```python
from build123d import *

# Parameters (mm, degrees)
SKETCH1_W               = 123
SKETCH1_H               = 20
SKETCH1_R               = 4.1
SKETCH1_R_2             = 4.5
BOSS_EXTRUDE1_DEPTH     = 8
FILLET1_R               = 5
FILLET2_R               = 5
CUT_EXTRUDE1_REACH      = 126.872
CUT_EXTRUDE1_END_RADIUS = 4.1
SKETCH2_R               = 1.5
CUT_EXTRUDE2_REACH      = 126.872
CUT_EXTRUDE2_END_RADIUS = 4.1
SKETCH3_R               = 1.5


with BuildPart() as part:
    # Sketch1 → Boss-Extrude1 (new body)
    with BuildSketch(Plane.XY):
        with Locations((-61.5, 10)):
            Rectangle(SKETCH1_W, SKETCH1_H)
        with Locations((-113.75, 10)):
            Circle(SKETCH1_R, mode=Mode.SUBTRACT)
        with Locations((-61.5, 10)):
            Circle(SKETCH1_R_2, mode=Mode.SUBTRACT)
        with Locations((-9.25, 10)):
            Circle(SKETCH1_R, mode=Mode.SUBTRACT)
    extrude(amount=BOSS_EXTRUDE1_DEPTH)

    # Fillet1
    fillet1_edges = [part.edges().sort_by_distance(p)[0] for p in [
        (-123, 20, 4),
    ]]
    fillet(fillet1_edges, radius=FILLET1_R)

    # Fillet2
    fillet2_edges = [part.edges().sort_by_distance(p)[0] for p in [
        (0, 0, 4),
        (-123, 0, 4),
        (0, 20, 4),
    ]]
    fillet(fillet2_edges, radius=FILLET2_R)

    # Cut-Extrude1: up to this cylinder (the profile starts outside it)
    cut_extrude1_end = Plane(origin=(-113.75, 10, 4), z_dir=(0, 0, -1)) * Cylinder(CUT_EXTRUDE1_END_RADIUS, 262.944, mode=Mode.PRIVATE)
    # Sketch2 → Cut-Extrude1 (cut, up to the surface)
    with BuildSketch(Plane.ZY.offset(123), mode=Mode.PRIVATE) as cut_extrude1_sk1:
        with Locations((4, 10)):
            Circle(SKETCH2_R)
    cut_extrude1_tool1 = extrude(cut_extrude1_sk1.sketch, amount=-CUT_EXTRUDE1_REACH, mode=Mode.PRIVATE) - cut_extrude1_end
    add(cut_extrude1_tool1.solids().sort_by_distance((-123, 10, 4))[0], mode=Mode.SUBTRACT)

    # Cut-Extrude2: up to this cylinder (the profile starts outside it)
    cut_extrude2_end = Plane(origin=(-9.25, 10, 4), z_dir=(0, 0, -1)) * Cylinder(CUT_EXTRUDE2_END_RADIUS, 262.944, mode=Mode.PRIVATE)
    # Sketch3 → Cut-Extrude2 (cut, up to the surface)
    with BuildSketch(Plane(origin=(0, 0, 0), x_dir=(0, 0, -1), z_dir=(1, 0, 0)), mode=Mode.PRIVATE) as cut_extrude2_sk1:
        with Locations(Location((-4, 10, 0), (0, 0, 180))):
            Circle(SKETCH3_R)
    cut_extrude2_tool1 = extrude(cut_extrude2_sk1.sketch, amount=-CUT_EXTRUDE2_REACH, mode=Mode.PRIVATE) - cut_extrude2_end
    add(cut_extrude2_tool1.solids().sort_by_distance((0, 10, 4))[0], mode=Mode.SUBTRACT)


solid = part.part
```
Geometry check sheet. Reference: the model listing, model coordinates, mm. A direction names the side the tool comes from. Give positions to 0.01 mm unless a question says otherwise; leave off trailing zeros. Order: outer loops, then holes, each group sorted by start corner. A loop starts at its lowest first (then second) coordinate and runs counter-clockwise, first axis right, second up. Notation, with made-up numbers: (-6.5, 57.5) - (21.5, 57.5) arc R11 ccw to (21.5, 71.5) - close; hole circle Ø10 at (-11.75, -8.75). An arc over 180 degrees is marked (long way). Answer in a Markdown table with one row per item. Add a question column.
Q1. Gauge pin test, flat ends, axial feed: pin 1 (2.5 mm diameter, centred on y = 10, z = 4, fed in from +X); pin 2 (4 mm diameter, centred on y = 17.5, z = 4.5, fed in from +X); pin 3 (1.8 mm diameter, centred on y = 10, z = 4, fed in from -X). Record the tip position at first contact, or that the pin passes through.
Q2. Material ranges on probe 1 along Z at (x, y) = (-119.9, 10); probe 2 along X at (y, z) = (8.5, 1); probe 3 along Y at (x, z) = (-113.75, 3.25), recorded low to high. Write a range as from..to.
Q3. Cross-section at D-D, the plane x = -61.5. Enter the section's corners in (y, z), then the cut area to 3 significant figures.
Q4. Mould release check, pull along X, two halves, no side actions. Record for faces 3 (the cylindrical face through (-109.84, 11.23, 3.94)), 4 (the cylindrical face through (-2.679, 10.575, 5.386)), 5 (the cylindrical face through (-2, 1, 4)): pulls with the +X half, pulls with the -X half, needs draft (parallel to the pull), parting line crosses it, or undercut.
Q5. Cross-section at A-A, the plane y = 10. Enter the section's corners in (x, z), then the cut area to 3 significant figures.
Q6. Tool access check on faces 1 (the flat face through (-62, 15, 8)), 2 (the cylindrical face through (-120.321, 9.425, 5.386)). Record the directions out of +Z, -Z, +X, -X, +Y, -Y that give a thin tool (end or side, any length) a straight path to the whole face; none if there is none.
Q7. Cross-section at B-B, the plane z = 1.5. Enter the section's corners in (x, y).
Q8. Cross-section at C-C, the plane x = -113.75. Enter the section's corners in (y, z).
Check values:
| question | item | result |
|---|---|---|
| 1 | pin 1 | stops at x = -13.15 |
| 1 | pin 2 | stops at x = -0.03 |
| 1 | pin 3 | stops at x = -109.75 |
| 2 | probe 1 | z = 0..2.5, 5.5..8 |
| 2 | probe 2 | x = -123..-117.57, -109.93..-65.74, -57.26..-13.07, -5.43..0 |
| 2 | probe 3 | y = 0..5.9, 14.1..20 |
| 3 | outline | (0, 0) - (5.5, 0) - (5.5, 8) - (0, 8) - close; (14.5, 0) - (20, 0) - (20, 8) - (14.5, 8) - close |
| 3 | area | 88.0 mm^2 |
| 4 | face 3 | undercut |
| 4 | face 4 | needs draft |
| 4 | face 5 | pulls with the +X half |
| 5 | outline | (-123, 0) - (-117.85, 0) - (-117.85, 2.5) - (-123, 2.5) - close; (-123, 5.5) - (-117.85, 5.5) - (-117.85, 8) - (-123, 8) - close; (-109.65, 0) - (-66, 0) - (-66, 8) - (-109.65, 8) - close; (-57, 0) - (-13.35, 0) - (-13.35, 8) - (-57, 8) - close; (-5.15, 0) - (0, 0) - (0, 2.5) - (-5.15, 2.5) - close; (-5.15, 5.5) - (0, 5.5) - (0, 8) - (-5.15, 8) - close |
| 5 | area | 750 mm^2 |
| 6 | face 1 | +Z, +X, -X, +Y, -Y |
| 6 | face 2 | -X |
| 7 | outline | (-123, 5) arc R5 ccw to (-118, 0) - (-5, 0) arc R5 ccw to (0, 5) - (0, 15) arc R5 ccw to (-5, 20) - (-118, 20) arc R5 ccw to (-123, 15) - close; hole circle Ø8.2 at (-113.75, 10); hole circle Ø9 at (-61.5, 10); hole circle Ø8.2 at (-9.25, 10) |
| 8 | outline | (0, 0) - (5.9, 0) - (5.9, 8) - (0, 8) - close; (14.1, 0) - (20, 0) - (20, 8) - (14.1, 8) - close |
